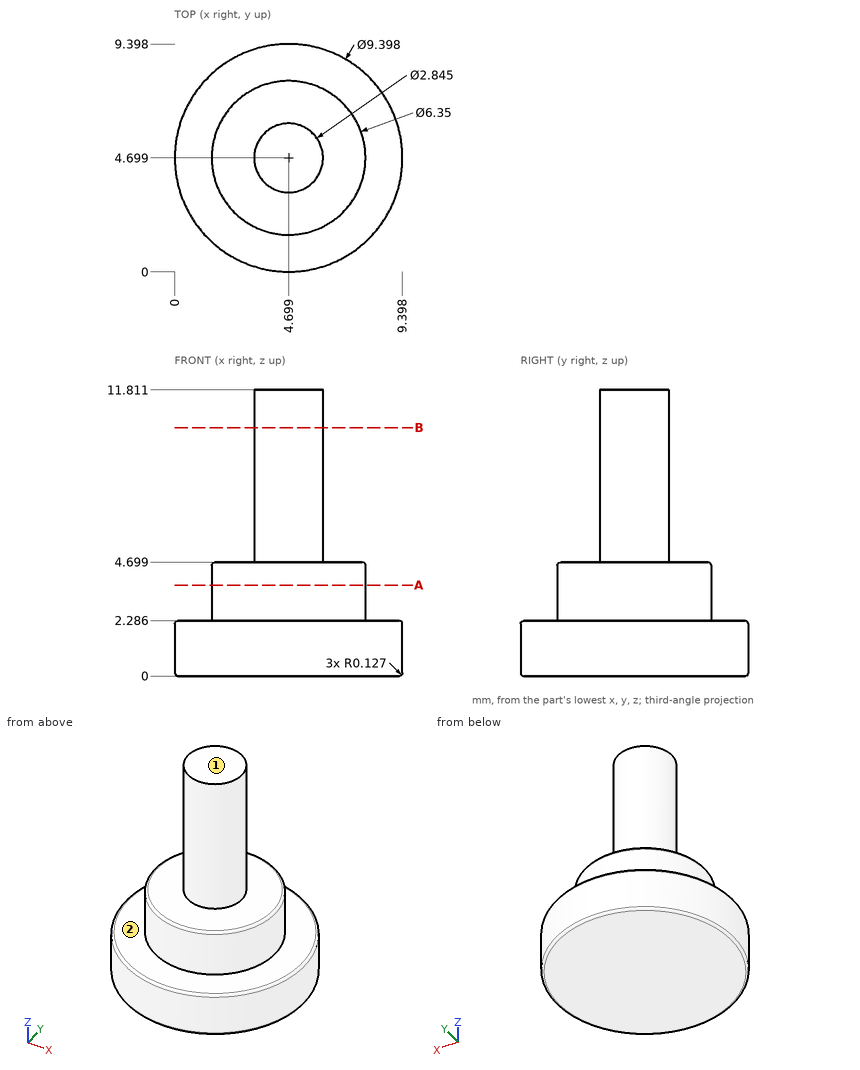
The figure shows three views and two pictorial views of one solid part (mm, origin at its lowest corner). Answer the questions. A direction names the side the tool comes from. Coordinates: 2 decimals unless noted, no trailing zeros. Write each loop counter-clockwise with the first axis right and the second up, starting at its lowest first coordinate (ties: lowest second). Pieces come first, ordered by that corner, then holes. Notation, with made-up numbers: (3.5, 9.5) -> (16.5, 9.5) arc R4 ccw to (16.5, 15.5) -> close; hole circle Ø2 at (21.25, 74). An arc over 180 degrees is marked (long way). Return JSON: item names as keys, results as strings.
(1) The part is cut by section B-B on z = 10.25. Give the vertices of the cut face in (x, y) (1 decimal).
Answers below:
{"outline": "circle Ø2.8 at (4.7, 4.7)"}
(2) The part is cut by section A-A on z = 3.75. Give the vertices of the cut face in (x, y) (3 decimals).
Answers below:
{"outline": "circle Ø6.35 at (4.699, 4.699)"}
(3) Each of these flat-tipped pins is pushed along its axis until it touches: P1, Ø1.5, axis at y = 1, z = 6, coming from the +X side; P2, Ø1.5, axis at y = 6.5, z = 7.5, coming from the -X side; P3, Ø3, axis at y = 3.5, z = 4, coming from the +X side. Where does it stop, or does it pass through?
Answers below:
{"P1": "through", "P2": "x = 3.74", "P3": "x = 7.87"}
(4) Which of the six approach directions +Z, -Z, +X, -X, +Y, -Y give full straight-line access (tool end or side, diameter ignored) to the marked faces 1 and 2?
Answers below:
{"face 1": "+Z, +X, -X, +Y, -Y", "face 2": "+Z"}
(5) Consider line 1 along X through (y, z) = (4.75, 4); line 2 along Z through (x, y) = (5.25, 7.5); line 3 along Z through (x, y) = (5.5, 8.75). Determine where each line is inside the solid, lowest interval first. Write a range as from..to.
Answers below:
{"line 1": "1.52..7.87", "line 2": "0..4.7", "line 3": "0..2.29"}
